Read the model definition and answer for the solid it produces. Units are mm, in the model's axes. A direction names the side the tool comes from. Give positions to 0.01 mm unless a question says otherwise; leave off trailing zeros. Write each loop counter-clockwise with the first axis right and the second up, starting at its lowest first coordinate (ties: lowest second). Pieces come first, ordered by that corner, then holes. Notation, with made-up numbers: (67, 51.25) -> (84, 51.25) arc R8 ccw to (84, 58.25) -> close; hole circle Ø1 at (-30.75, 9.5). An arc over 180 degrees is marked (long way). Write item = value, one per line.
from build123d import *

# Parameters (mm, degrees)
CROQUIS1_W               = 40.8
CROQUIS1_H               = 40.8
SALIENTE_EXTRUIR1_DEPTH  = 22.6
SALIENTE_EXTRUIR1_TAPER  = 2
CROQUIS2_W               = 28.1
CROQUIS2_H               = 28.1
SALIENTE_EXTRUIR2_DEPTH  = 0.75
REDONDEO1_R              = 1
CROQUIS3_R               = 7.5
SALIENTE_EXTRUIR3_DEPTH  = 9
CROQUIS4_R               = 5.8
SALIENTE_EXTRUIR4_DEPTH  = 3
CROQUIS7_R               = 2.5
SALIENTE_EXTRUIR7_DEPTH  = 5
REDONDEO5_R              = 1
CROQUIS16_R              = 11.5
SALIENTE_EXTRUIR12_DEPTH = 4.5
CROQUIS17_R              = 8.836056804
SALIENTE_EXTRUIR13_DEPTH = 0.5
REDONDEO9_R              = 20


with BuildPart() as part:
    # Croquis1 → Saliente-Extruir1 (new body)
    with BuildSketch(Plane.XY):
        Rectangle(CROQUIS1_W, CROQUIS1_H)
    extrude(amount=SALIENTE_EXTRUIR1_DEPTH, taper=SALIENTE_EXTRUIR1_TAPER)

    # Croquis2 → Saliente-Extruir2 (add, symmetric)
    with BuildSketch(Plane.XY.offset(22.6)):
        Rectangle(CROQUIS2_W, CROQUIS2_H)
    extrude(amount=SALIENTE_EXTRUIR2_DEPTH, both=True)

    # Redondeo1
    # the kernel refuses this fillet: 1 mm, written as the material it takes off along each edge
    with BuildSketch(Plane(origin=(14.05, 16.470614591, 23.35), x_dir=(0, 0, -1), z_dir=(0, -1, 0)), Plane(origin=(-16.470614591, 14.05, 23.35), x_dir=(0, 0, -1), z_dir=(1, 0, 0)), Plane(origin=(16.470614591, -14.05, 23.35), x_dir=(0, 0, -1), z_dir=(-1, 0, 0)), Plane(origin=(-14.05, -16.470614591, 23.35), x_dir=(0, 0, -1), z_dir=(0, 1, 0))) as redondeo1_piece_1:
        with BuildLine():
            CenterArc((1, -0.968245837), REDONDEO1_R, 104.477512186, 75.522487814)
            Line((0, -0.968245837), (-0.02, -0.968245837))
            Line((-0.02, -0.968245837), (-0.02, 0))
            Line((-0.02, 0), (0, 0.02))
            ThreePointArc((0, 0.02), (0.375, 0.02), (0.745, 0.019364917))
            Line((0.745, 0.019364917), (0.75, 0))
        make_face()
    extrude(amount=32.941229183, mode=Mode.SUBTRACT)

    # Croquis3 → Saliente-Extruir3 (add)
    with BuildSketch(Plane.XY.offset(23.35)):
        Circle(CROQUIS3_R)
    extrude(amount=SALIENTE_EXTRUIR3_DEPTH)

    # Croquis4 → Saliente-Extruir4 (add)
    with BuildSketch(Plane.XY.offset(32.35)):
        Circle(CROQUIS4_R)
    extrude(amount=SALIENTE_EXTRUIR4_DEPTH)

    # Croquis7 → Saliente-Extruir7 (add)
    with BuildSketch(Plane(origin=(0, 0, 0), x_dir=(-1, 0, 0), z_dir=(0, 0, -1))):
        with Locations(Location((-9.4, 11.9, 0), (0, 0, 180))):
            Circle(CROQUIS7_R)
    extrude(amount=SALIENTE_EXTRUIR7_DEPTH)

    # Redondeo5
    redondeo5_edges = [part.edges().sort_by_distance(p)[0] for p in [
        (-19.610790609, 0, 22.6),
        (0, -19.610790609, 22.6),
        (19.610790609, 0, 22.6),
        (0, -20.4, 0),
        (-20.4, 0, 0),
        (0, 20.4, 0),
        (20.4, 0, 0),
        (20.005395305, -20.005395305, 11.3),
        (-20.005394843, -20.005394843, 11.300013228),
        (-20.005395305, 20.005395305, 11.3),
        (20.005394843, 20.005394843, 11.300013228),
        (0, 19.610790609, 22.6),
    ]]
    fillet(redondeo5_edges, radius=REDONDEO5_R)

    # Croquis16 → Saliente-Extruir12 (add)
    with BuildSketch(Plane.XY.offset(35.35)):
        Circle(CROQUIS16_R)
    extrude(amount=SALIENTE_EXTRUIR12_DEPTH)

    # Croquis17 → Saliente-Extruir13 (add)
    with BuildSketch(Plane.XY.offset(39.85)):
        Circle(CROQUIS17_R)
    extrude(amount=SALIENTE_EXTRUIR13_DEPTH)

    # Redondeo9
    # the kernel refuses this fillet: 20 mm, written as the material it takes off along each edge
    with BuildSketch(Plane(origin=(0, 0, 40.35), x_dir=(1, 0, 0), z_dir=(0, -1, 0))) as redondeo9_piece_1:
        with BuildLine():
            CenterArc((4.391959596, -20), REDONDEO9_R, 77.161431859, 12.838568141)
            Line((4.391959596, 0), (4.391959596, 0.4))
            Line((4.391959596, 0.4), (8.836056804, 0.4))
            Line((8.836056804, 0.4), (9.236056804, 0))
            ThreePointArc((9.236056804, 0), (9.236056804, -0.25), (8.924938748, -0.11))
            Line((8.924938748, -0.11), (8.836056804, -0.5))
        make_face()
    revolve(axis=Axis((0, 0, 40.35), (0, 0, 1)), mode=Mode.SUBTRACT)


solid = part.part
(1) Given P1, Ø1, axis at x = -9.5, z = 15, coming from the +Y side; P2, Ø3, axis at y = 5.5, z = 17.5, coming from the -X side; P3, Ø5, axis at y = 6, z = 28, coming from the +X side, each flat-ended and moving along its own axis, determine where each tip first touches the part or whether it passes through.
Checks:
P1 = 19.89
P2 = -19.84
P3 = 6.63
(2) Consider L1, parallel to Y at x = 0, z = 33.5; L2, parallel to Z at x = -12, y = -10.5; L3, parallel to Z at x = 0, y = 17. Determine where each line is inside the solid, lowest interval first.
Checks:
L1 = -5.8 to 5.8
L2 = 0 to 23.35
L3 = 0 to 22.6
(3) The part is cut by section B-B on z = 26.5. Determine the outline of the cut face in (x, y).
Checks:
outline = circle Ø15 at (0, 0)
(4) A tool of negligible diameter and unlimited length cuts with its end or side. For faces 1 (the flat face through (0, 0, 40.35)), 2 (the flat face through (2, -6, 32.35)), 3 (the cylindrical face through (-19.71, 19.7, 11.49)), 4 (the flat face through (16, 0, 22.6)), 5 (the cylindrical face through (7.56, 10.21, -2.46)), from which of +Z, -Z, +X, -X, +Y, -Y can it reach the whole face along a straight path? Write none if from no direction.
Checks:
face_1 = +Z, +X, -X, +Y, -Y
face_2 = none
face_3 = +Z, -X, +Y
face_4 = +Z
face_5 = -Z
(5) For a pull along Z with two mould halves and no side action, classify faces 6 (the cylindrical face through (-1.5, 11.4, 37.6)), 7 (the flat face through (-6, -6, 23.35)), 8 (the flat face through (3.4, -8.5, 39.85)) as released by +Z, released by -Z, zero draft, split by the parting line, or undercut.
Checks:
face_6 = zero draft
face_7 = undercut
face_8 = released by +Z
